Geometry: final body of the model. Coordinates: model frame, mm. Give positions to 0.01 mm unless a question says otherwise; leave off trailing zeros. Write each loop counter-clockwise with the first axis right and the second up, starting at its lowest first coordinate (ties: lowest second). Pieces come first, ordered by that corner, then holes. Notation, with made-up numbers: M 21.25,56 L 54.25,56 A25 ccw 54.25,89 Z; hole C 3.25,-10.5 d7. An arc over 180 degrees is marked long. Use a Markdown table: item, result. Add a question column.
(1) Cut plane A-A (x = -22). Output: boundary loops of the cut face in (y, z).
(2) Draft query along Z for faces 1 (the cylindrical face through (-23.11, -1.52, 23.01)), 2 (the flat face through (-25, -1, 0)), 3 (the flat face through (0, -1, 25)). Return one class per face: released by +Z, released by -Z, zero draft, split by the parting line, or undercut.
(3) Cut plane B-B (z = 22). Output: boundary loops of the cut face in (x, y), plus the area to 3 significant figures.
(4) Pin query (flat end, axial travel): pin 1 Ø4 at (x, z) = (15, -11.5) entering from +Y. Return the tip coordinate at first contact, or that it passes through.
(5) Material intervals for L1, parallel to Z at x = -22, y = -0.95; L2, parallel to Z at x = -21, y = -0.55, sorted ascending.
```python
from build123d import *

# Parameters (mm, degrees)
F0_W     = 50
F0_H     = 50
F1_DEPTH = 3
F2_R     = 1.5
F3_DEPTH = 25


with BuildPart() as f1:
    # F0 (on Front) → F1 (new body)
    with BuildSketch(Plane.XZ):
        Rectangle(F0_W, F0_H)
    extrude(amount=F1_DEPTH)

    # F2 (on face) → F3 (cut)
    with BuildSketch(Plane.XZ.offset(3)):
        with Locations((-22, 22)):
            Circle(F2_R)
    extrude(amount=-F3_DEPTH, mode=Mode.SUBTRACT)


solid = f1.part
```
Answer list:
| question | item | result |
|---|---|---|
| 1 | outline | M -3,-25 L 0,-25 L 0,20.5 L -3,20.5 Z; M -3,23.5 L 0,23.5 L 0,25 L -3,25 Z |
| 2 | face 1 | undercut |
| 2 | face 2 | zero draft |
| 2 | face 3 | released by +Z |
| 3 | outline | M -25,-3 L -23.5,-3 L -23.5,0 L -25,0 Z; M -20.5,-3 L 25,-3 L 25,0 L -20.5,0 Z |
| 3 | area | 141 mm² |
| 4 | pin 1 | y = 0 |
| 5 | L1 | -25 to 20.5, 23.5 to 25 |
| 5 | L2 | -25 to 20.88, 23.12 to 25 |
